Geometry: final body of the model. Coordinates: model frame, mm. A direction names the side the tool comes from. Coordinates: 2 decimals unless noted, no trailing zeros. Loops run counter-clockwise (first coordinate to the right, second up) from the corner with the lowest first, then second, coordinate; pieces in that order, holes last. Notation, with made-up numbers: (39.25, 1) -> (49.25, 1) arc R19 cw to (49.25, 33) -> close; hole circle Ø10 at (33.25, 89). An arc over 180 degrees is marked (long way). One line per item, written item: value. Start each with the question number.
Item 1: Mould query, pull axis Z, two halves, no side actions, for faces 1 (the cylindrical face through (35.722, -36.975, 79.125)), 2 (the cylindrical face through (105.7, -37, -69.7)), 3 (the flat face through (50.08, -45.31, -45)). Classes: +Z half, -Z half, draft (parallel to the pull), parting line (faces both ways), or undercut.
Item 2: Set-up query: faces 4 (the cylindrical face through (76.98, -36.98, -73.81)), 5 (the flat face through (-12.18, -36.98, 36.05)), 6 (the cylindrical face through (89.061, -36.975, -63.556)). Return all of +Z, -Z, +X, -X, +Y, -Y with unobstructed straight access to the full face (end or side cutting, diameter ignored); none if empty.
Item 3: Section query B-B on x = -39.5. Return loops of the section in (y, z).
Item 4: Section query D-D on z = 37. Return loops of the section in (x, y), then the cut area to 3 significant figures.
Item 5: Ray query, probe 1 along X at (y, z) = (-8.5, -28.5); probe 2 along X at (y, z) = (-65, -39); probe 3 along X at (y, z) = (-19.5, -51). Return the intervals inside material, ascending. Write a range as from..to.
Item 6: Section query A-A on x = -84.5. Return loops of the section in (y, z).
Item 7: Contact query for flat-ended pins moving along their axis: pin 1 Ø12 at (y, z) = (-61, -34.5) entering from -X; pin 2 Ø6 at (x, y) = (-92.5, -10) entering from +Z; pin 3 Ø1.4 at (x, y) = (-72.5, -59) entering from +Z. Output: stop coordinate, or through.
Item 8: Section query C-C on x = 35. Return loops of the section in (y, z).
from build123d import *

# Parameters (mm, degrees)
F1_DEPTH      = 75
F3_DEPTH      = 30
F3_DEPTH_BACK = 90
F4_W          = 60.3201809678
F4_H          = 11.285925284
F5_DEPTH      = 25
F5_DEPTH_BACK = 10


with BuildPart() as f1:
    # F0 (on Front) → F1 (new body)
    with BuildSketch(Plane.XZ):
        with BuildLine():
            Line((31.9086386453, 77.6905462364), (-57.5139995569, -6.7641266773))
            ThreePointArc((-57.5139995569, -6.7641266773), (-57.9219339607, -7.0245091068), (-58.3971183008, -7.1162115075))
            ThreePointArc((-58.3971183008, -7.1162115075), (-69.4887089259, -0.8420637784), (-69.7767442137, 11.8978478381))
            ThreePointArc((-69.7767442137, 11.8978478381), (-69.8049165196, 13.1707831552), (-70.9122465225, 13.7992561182))
            Line((-70.9122465225, 13.7992561182), (-73.6895077641, 13.7992561182))
            ThreePointArc((-73.6895077641, 13.7992561182), (-74.0062961207, 13.726942606), (-74.2603264098, 13.5243278998))
            Line((-74.2603264098, 13.5243278998), (-75.8568685996, 11.5219015441))
            ThreePointArc((-75.8568685996, 11.5219015441), (-77.5081657489, 0.4349594479), (-71.8249073519, -9.226698863))
            ThreePointArc((-71.8249073519, -9.226698863), (-69.2584995586, -14.5376929324), (-71.5152183851, -19.9874935806))
            Line((-71.5152183851, -19.9874935806), (-116.5955893061, -62.5633788748))
            ThreePointArc((-116.5955893061, -62.5633788748), (-116.2574535182, -71.2949238612), (-108.6162978034, -75.5336681331))
            Line((-108.6162978034, -75.5336681331), (-56.4006080373, -75.5336681323))
            ThreePointArc((-56.4006080373, -75.5336681323), (-54.2860073929, -75.2694967603), (-52.3013870442, -74.4932207332))
            Line((-52.3013870442, -74.4932207332), (9.3968417232, -41.0165915738))
            ThreePointArc((9.3968417232, -41.0165915738), (13.3164182298, -39.9780216691), (17.2759733413, -40.8518813589))
            Line((17.2759733413, -40.8518813589), (58.3416101428, -60.9595264103))
            ThreePointArc((58.3416101428, -60.9595264103), (58.4992740431, -61.0453458085), (58.6489560893, -61.1444324351))
            Line((58.6489560893, -61.1444324351), (74.0206310135, -72.3025880245))
            ThreePointArc((74.0206310135, -72.3025880245), (77.0205825857, -73.8239393845), (80.345354257, -74.3339518648))
            Line((80.345354257, -74.3339518648), (84.008830193, -74.3106924806))
            Line((84.008830193, -74.3106924806), (94.6409664598, -74.2431891184))
            ThreePointArc((94.6409664598, -74.2431891184), (105.8729254369, -69.5279758333), (110.516733495, -58.2663069736))
            Line((110.516733495, -58.2663069736), (110.516733495, -57.3599657599))
            ThreePointArc((110.516733495, -57.3599657599), (108.6798338491, -49.9220331846), (103.5915117273, -44.1943792767))
            Line((103.5915117273, -44.1943792767), (80.0608191671, -28.0158812776))
            ThreePointArc((80.0608191671, -28.0158812776), (78.5255862483, -27.6803464363), (77.1934165925, -28.5139217195))
            Line((77.1934165925, -28.5139217195), (75.6298542432, -30.6832325702))
            ThreePointArc((75.6298542432, -30.6832325702), (74.1211917974, -36.9659668973), (77.4545705219, -42.5010729739))
            Line((77.4545705219, -42.5010729739), (96.61347436, -56.7622144645))
            ThreePointArc((96.61347436, -56.7622144645), (97.7016607764, -59.4192137179), (95.8614861172, -61.6231991836))
            ThreePointArc((95.8614861172, -61.6231991836), (88.9594846076, -63.5579741018), (81.9860902339, -61.8988328387))
            Line((81.9860902339, -61.8988328387), (17.2686592302, -27.626202898))
            ThreePointArc((17.2686592302, -27.626202898), (13.2025716128, -26.6269144318), (9.1467925766, -27.6672520504))
            Line((9.1467925766, -27.6672520504), (-49.2817682282, -59.3698033465))
            ThreePointArc((-49.2817682282, -59.3698033465), (-69.8161964781, -54.7329590263), (-67.9299516201, -33.7661960635))
            Line((-67.9299516201, -33.7661960635), (39.9862620913, 69.185022562))
            ThreePointArc((39.9862620913, 69.185022562), (41.616957342, 72.8737890727), (40.1616811978, 76.6352165564))
            Line((40.1616811978, 76.6352165564), (39.3396363558, 77.4969058889))
            ThreePointArc((39.3396363558, 77.4969058889), (35.6640993707, 79.1272730212), (31.9086386453, 77.6905462364))
        make_face()
    extrude(amount=F1_DEPTH)

    # F2 (on face) → F3 (cut, two sides)
    with BuildSketch(Plane(origin=(-23.7385230795, 0, 25.1349189755), x_dir=(0.7270133187, 0, 0.686623357), z_dir=(-0.686623357, 0, 0.7270133187))) as f3_sk:
        Polygon((-46.4578510571, -24.0551400103), (-143.9990401268, -21.0843849927), (-143.4555607145, -53.2556629783), (-46.4578510571, -50.6537381076), align=None)
        with BuildLine():
            Line((-18.389185364, -24.9100109652), (-46.4578510571, -24.0551400103))
            Line((-46.4578510571, -24.0551400103), (-46.4578510571, -50.6537381076))
            Line((-46.4578510571, -50.6537381076), (-18.4254588112, -49.9017803673))
            ThreePointArc((-18.4254588112, -49.9017803673), (-11.5283625374, -46.8809946351), (-8.6936083649, -39.905376223))
            Line((-8.6936083649, -39.905376223), (-8.6936083649, -34.905376223))
            ThreePointArc((-8.6936083649, -34.905376223), (-11.5157176577, -27.9427700303), (-18.389185364, -24.9100109652))
        make_face()
    extrude(amount=F3_DEPTH, mode=Mode.SUBTRACT)
    extrude(f3_sk.sketch, amount=-F3_DEPTH_BACK, mode=Mode.SUBTRACT)

    # F4 (on face) → F5 (cut, two sides)
    with BuildSketch(Plane(origin=(-7.6435291417, 0, -14.433370614), x_dir=(0.8837288425, 0, -0.4679992873), z_dir=(0.4679992873, 0, 0.8837288425))) as f5_sk:
        with Locations((58.3499459846, -37.2247295454)):
            Rectangle(F4_W, F4_H)
        with BuildLine():
            ThreePointArc((3.452683799, -39.8676921874), (4.3313634554, -41.989012531), (6.452683799, -42.8676921874))
            Line((6.452683799, -42.8676921874), (28.1898555007, -42.8676921874))
            Line((28.1898555007, -42.8676921874), (28.1898555007, -31.5817669034))
            Line((28.1898555007, -31.5817669034), (6.452683799, -31.5817669034))
            ThreePointArc((6.452683799, -31.5817669034), (4.3313634554, -32.4604465598), (3.452683799, -34.5817669034))
            Line((3.452683799, -34.5817669034), (3.452683799, -39.8676921874))
        make_face()
    extrude(amount=-F5_DEPTH, mode=Mode.SUBTRACT)
    extrude(f5_sk.sketch, amount=F5_DEPTH_BACK, mode=Mode.SUBTRACT)


solid = f1.part
Reply:
1. face 1: +Z half
1. face 2: -Z half
1. face 3: undercut
2. face 4: -Z, +Y, -Y
2. face 5: +Z, +Y, -Y
2. face 6: +Y, -Y
3. outline: (-75, -67.55) -> (-51.42, -67.55) -> (-51.17, -54.06) -> (-75, -54.06) -> close; (-75, -6.64) -> (-50.3, -6.64) -> (-49.99, 10.25) -> (-75, 10.25) -> close; (-24.81, 10.25) -> (-24.46, -6.64) -> (0, -6.64) -> (0, 10.25) -> close; (-23.46, -54.06) -> (-23.18, -67.55) -> (0, -67.55) -> (0, -54.06) -> close
4. outline: (-11.18, -75) -> (6.25, -75) -> (6.25, 0) -> (-11.18, 0) -> close
4. area: 1,310 mm²
5. probe 1: x = -80.53..-62.41, 7.61..18.92, 77.2..80.76
5. probe 2: x = -91.65..-71.57, -11.74..38.75, 74.7..96.04
5. probe 3: x = -104.35..-71.84, -33.86..-9, 38..61.41, 88.87..109.2
6. outline: (-75, -75.53) -> (-52.45, -75.53) -> (-51.65, -32.25) -> (-75, -32.25) -> close; (-22.92, -32.25) -> (-22.02, -75.53) -> (0, -75.53) -> (0, -32.25) -> close
7. pin 1: stops at x = -93.23
7. pin 2: stops at z = -36.97
7. pin 3: stops at z = 13.8
8. outline: (-75, -49.53) -> (-42.87, -49.53) -> (-42.87, -37.02) -> (-75, -37.02) -> close; (-75, 64.43) -> (0, 64.43) -> (0, 79.1) -> (-75, 79.1) -> close; (-31.58, -49.53) -> (0, -49.53) -> (0, -37.02) -> (-31.58, -37.02) -> close
